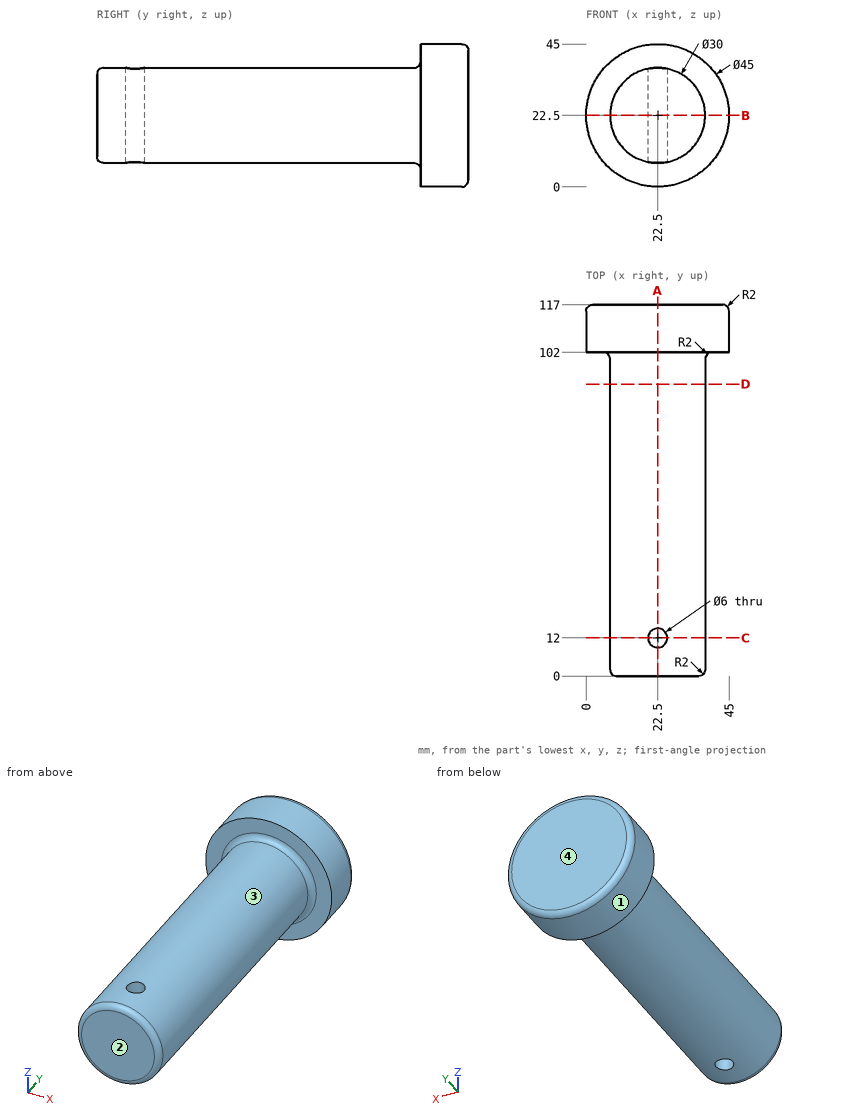
Can you work these out from the drawing? Everything is in mm from the part's minimum corner. A direction names the side the tool comes from. Give positions to 0.01 mm unless a question says otherwise; leave off trailing zeros. Write each loop counter-clockwise with the first axis right and the second up, starting at its lowest first coordinate (ties: lowest second). Pieces come first, ordered by that corner, then holes. Notation, with made-up numbers: (58.25, 1) -> (91.25, 1) arc R23 cw to (91.25, 24) -> close; hole circle Ø11 at (27.5, -27.75). An arc over 180 degrees is marked (long way). Write each question's results on one line, items separated by ' | '. Start each with the question number.
Q1. I'm going to push flat-ended pins straight in: pin 1 Ø12 at (y, z) = (90, 22) entering from +X; pin 2 Ø12 at (y, z) = (16, 31.5) entering from -X; pin 3 Ø4 at (x, y) = (8.5, 91.5) entering from +Z. Where does each tip first touch, or does it pass through?
Q2. Suppose I cut it at C-C, the plane y = 12. List the corners of the cut face in (x, z) for me, and give its area (3 significant figures).
Q3. Suppose I cut it at D-D, the plane y = 92. List the corners of the cut face in (x, z) for me, and give its area (3 significant figures).
Q4. Suppose I cut it at A-A, the plane x = 22.5. List the corners of the cut face in (y, z) for me.
Q5. We'd pull the mould along X, two halves only. Please class the marked faces 1 and 2: +X half, -X half, draft (parallel to the pull), parting line (faces both ways), or undercut.
Q6. I need wall thicknesses on probe 1 along X at (y, z) = (12, 23); probe 2 along Y at (x, z) = (22.5, 27.5); probe 3 along Y at (x, z) = (5.5, 33.5). Which ranges of each line are inside material? Lowest first, please.
Q7. Which directions (+Z, -Z, +X, -X, +Y, -Y) give clear straight access to the entire face, cutting with the end or side of a thin tool? Please do the marked faces 3 and 4.
Q8. Suppose I cut it at B-B, the plane z = 22.5. List the corners of the cut face in (x, y) for me.
Outcome:
1) pin 1: x = 37.5 | pin 2: x = 7.8 | pin 3: z = 31.5
2) outline: (19.5, 7.8) -> (19.5, 37.2) arc R15 ccw to start; (25.5, 7.8) arc R15 ccw to (25.5, 37.2) -> close | area: 528 mm2
3) outline: circle Ø30 at (22.5, 22.5) | area: 707 mm2
4) outline: (0, 9.5) arc R2 ccw to (2, 7.5) -> (9, 7.5) -> (9, 37.5) -> (2, 37.5) arc R2 ccw to (0, 35.5) -> close; (15, 7.5) -> (100, 7.5) arc R2 cw to (102, 5.5) -> (102, 0) -> (115, 0) arc R2 ccw to (117, 2) -> (117, 43) arc R2 ccw to (115, 45) -> (102, 45) -> (102, 39.5) arc R2 cw to (100, 37.5) -> (15, 37.5) -> close
5) face 1: parting line | face 2: draft
6) probe 1: 7.51 to 19.5, 25.5 to 37.49 | probe 2: 0 to 9, 15 to 117 | probe 3: 102 to 117
7) face 3: -Y | face 4: +Z, -Z, +X, -X, +Y
8) outline: (0, 102) -> (5.5, 102) arc R2 cw to (7.5, 100) -> (7.5, 2) arc R2 ccw to (9.5, 0) -> (35.5, 0) arc R2 ccw to (37.5, 2) -> (37.5, 100) arc R2 cw to (39.5, 102) -> (45, 102) -> (45, 115) arc R2 ccw to (43, 117) -> (2, 117) arc R2 ccw to (0, 115) -> close; hole circle Ø6 at (22.5, 12)
